```python
from build123d import *

# Parameters (mm, degrees)
SKETCH1_R                = 4
BOSS_EXTRUDE1_DEPTH      = 28
SKETCH2_W                = 40.5
SKETCH2_H                = 38
CUT_EXTRUDE1_DEPTH       = 23
SKETCH3_R                = 9.65
CUT_EXTRUDE2_DEPTH       = 5
CUT_EXTRUDE3_START       = -5
SKETCH4_R                = 9.65
CUT_EXTRUDE3_DEPTH       = 5
SKETCH8_R                = 1.15
CUT_EXTRUDE7_DEPTH       = 76.219678276
CHAMFER1_SIZE            = 23
CHAMFER1_SIZE2           = 43.5
SKETCH9_R                = 2.2
CUT_EXTRUDE8_DEPTH       = 97.701654612
CUT_EXTRUDE9_DEPTH       = 3
CUT_EXTRUDE9_DEPTH_BACK  = 4
CHAMFER2_SIZE            = 3
SKETCH15_R               = 1.7
CUT_EXTRUDE11_DEPTH      = 76.219678334
SKETCH16_W               = 26
SKETCH16_H               = 38
CUT_EXTRUDE12_DEPTH      = 67.075411499
FILLET6_R                = 1.5
CUT_EXTRUDE13_START      = -17
CUT_EXTRUDE13_DEPTH      = 17
BOSS_EXTRUDE3_DEPTH      = 4.5
BOSS_EXTRUDE3_DEPTH_BACK = 4.5
SKETCH21_R               = 1.65
SKETCH22_R               = 4.5
CUT_EXTRUDE14_DEPTH      = 7
CHAMFER4_SIZE            = 8.5
CHAMFER4_SIZE2           = 10
FILLET1_R                = 5
FILLET2_R                = 6
FILLET4_R                = 12
CUT_EXTRUDE15_DEPTH      = 3.8
CUT_EXTRUDE18_REACH      = 77.22
SKETCH26_R               = 3.15


with BuildPart() as part:
    # Sketch1 → Boss-Extrude1 (new body)
    with BuildSketch(Plane.XY):
        with BuildLine():
            Line((-55, -23.6), (34.5, -23.6))
            Line((34.5, -23.6), (34.5, 19.4))
            Line((34.5, 19.4), (-28.5, 19.4))
            Line((-28.5, 19.4), (-28.5, 12.180409823))
            ThreePointArc((-28.5, 12.180409823), (-20.217668105, -2.285689125), (-33, -12.985083113))
            Line((-33, -12.985083113), (-36, -12.985083113))
            ThreePointArc((-36, -12.985083113), (-41.689100041, -11.672468641), (-46.228019527, -8))
            Line((-46.228019527, -8), (-55, -8))
            Line((-55, -8), (-55, -23.6))
        make_face()
        Circle(SKETCH1_R, mode=Mode.SUBTRACT)
        with BuildLine():
            Line((-23, 11.35), (-20, 11.35))
            ThreePointArc((-20, 11.35), (-18.35, 13), (-20, 14.65))
            Line((-20, 14.65), (-23, 14.65))
            ThreePointArc((-23, 14.65), (-24.65, 13), (-23, 11.35))
        make_face(mode=Mode.SUBTRACT)
        with BuildLine():
            Line((-23, -14.65), (-20, -14.65))
            ThreePointArc((-20, -14.65), (-18.35, -13), (-20, -11.35))
            Line((-20, -11.35), (-23, -11.35))
            ThreePointArc((-23, -11.35), (-24.65, -13), (-23, -14.65))
        make_face(mode=Mode.SUBTRACT)
        with BuildLine():
            Line((-46, -11.35), (-49, -11.35))
            ThreePointArc((-49, -11.35), (-50.65, -13), (-49, -14.65))
            Line((-49, -14.65), (-46, -14.65))
            ThreePointArc((-46, -14.65), (-44.35, -13), (-46, -11.35))
        make_face(mode=Mode.SUBTRACT)
    extrude(amount=BOSS_EXTRUDE1_DEPTH)

    # Sketch2 → Cut-Extrude1 (cut)
    with BuildSketch(Plane.XY.offset(28)):
        with Locations((-34.75, 0.4)):
            Rectangle(SKETCH2_W, SKETCH2_H)
    extrude(amount=-CUT_EXTRUDE1_DEPTH, mode=Mode.SUBTRACT)

    # Sketch3 → Cut-Extrude2 (cut)
    with BuildSketch(Plane.XY.offset(28)):
        Circle(SKETCH3_R)
    extrude(amount=-CUT_EXTRUDE2_DEPTH, mode=Mode.SUBTRACT)

    # Sketch4 → Cut-Extrude3 (cut)
    with BuildSketch(Plane(origin=(0, 0, 0), x_dir=(-1, 0, 0), z_dir=(0, 0, -1)).offset(CUT_EXTRUDE3_START)):
        with Locations(Location((0, 0, 0), (0, 0, 180))):
            Circle(SKETCH4_R)
    extrude(amount=CUT_EXTRUDE3_DEPTH, mode=Mode.SUBTRACT)

    # Sketch8 → Cut-Extrude7 (cut, through all)
    with BuildSketch(Plane.XZ.offset(23.6)):
        with Locations(Location((3.375, 15.5, 0), (0, 0, 270))):
            Circle(SKETCH8_R)
    extrude(amount=-CUT_EXTRUDE7_DEPTH, mode=Mode.SUBTRACT)

    # Chamfer1
    chamfer1_edges = [part.edges().sort_by_distance(p)[0] for p in [
        (-55, -21.1, 28),
    ]]
    chamfer1_side = [part.faces().sort_by_distance(p)[0] for p in [
        (-55, -18.958031088, 10.841968912),
    ]]
    chamfer(chamfer1_edges, length=CHAMFER1_SIZE, length2=CHAMFER1_SIZE2, reference=chamfer1_side[0])

    # Sketch9 → Cut-Extrude8 (cut, through all)
    with BuildSketch(Plane(origin=(34.5, 0, 0), x_dir=(0, 0, -1), z_dir=(1, 0, 0))):
        with Locations((-8, 13)):
            Circle(SKETCH9_R)
        with Locations((-23, 13)):
            Circle(SKETCH9_R)
    extrude(amount=-CUT_EXTRUDE8_DEPTH, mode=Mode.SUBTRACT)

    # Sketch10 → Cut-Extrude9 (cut, two sides: drawn at the far end of the back side and taken through both)
    with BuildSketch(Plane.ZY.offset(14.5).offset(-CUT_EXTRUDE9_DEPTH_BACK)):
        Polygon((5.1, 14.674315781), (5.1, 11.325684219), (8, 9.651368439), (10.9, 11.325684219), (10.9, 14.674315781), (8, 16.348631561), align=None)
        Polygon((25.9, 11.325684219), (25.9, 14.674315781), (23, 16.348631561), (20.1, 14.674315781), (20.1, 11.325684219), (23, 9.651368439), align=None)
    extrude(amount=CUT_EXTRUDE9_DEPTH + CUT_EXTRUDE9_DEPTH_BACK, mode=Mode.SUBTRACT)

    # Chamfer2
    chamfer2_edges = [part.edges().sort_by_distance(p)[0] for p in [
        (-14.5, -18.6, 15.706896552),
    ]]
    chamfer(chamfer2_edges, length=CHAMFER2_SIZE)

    # Sketch15 → Cut-Extrude11 (cut, through all)
    with BuildSketch(Plane.XZ.offset(23.6)):
        with Locations(Location((-20.625, 15, 0), (0, 0, 270))):
            Circle(SKETCH15_R)
        with Locations(Location((29.375, 15, 0), (0, 0, 270))):
            Circle(SKETCH15_R)
    extrude(amount=-CUT_EXTRUDE11_DEPTH, mode=Mode.SUBTRACT)

    # Sketch16 → Cut-Extrude12 (cut, through all)
    with BuildSketch(Plane.XY.offset(28)):
        with Locations((21.5, 0.4)):
            Rectangle(SKETCH16_W, SKETCH16_H)
    extrude(amount=-CUT_EXTRUDE12_DEPTH, mode=Mode.SUBTRACT)

    # Fillet6
    fillet6_edges = [part.edges().sort_by_distance(p)[0] for p in [
        (8.5, -18.6, 14),
    ]]
    fillet(fillet6_edges, radius=FILLET6_R)

    # Sketch17 → Cut-Extrude13 (cut)
    with BuildSketch(Plane.XY.offset(28).offset(CUT_EXTRUDE13_START)):
        with BuildLine():
            Line((0, 4), (0, 15.733500455))
            Line((0, 15.733500455), (8.5, 15.733500455))
            Line((8.5, 15.733500455), (8.5, -8.907477288))
            Line((8.5, -8.907477288), (0, -4))
            ThreePointArc((0, -4), (4, 0), (0, 4))
        make_face()
    extrude(amount=CUT_EXTRUDE13_DEPTH, mode=Mode.SUBTRACT)

    # Sketch20 → Cut-Revolve1 (revolve, cut)
    with BuildSketch(Plane.XY.offset(15.5), mode=Mode.PRIVATE) as cut_revolve1_sk:
        Polygon((3.375, -11.8), (7.375, -3.8), (3.375, -3.8), align=None)
    revolve(cut_revolve1_sk.sketch.rotate(Axis((3.375, -3.8, 15.5), (0, -1, 0)), 270), axis=Axis((3.375, -3.8, 15.5), (0, -1, 0)), mode=Mode.SUBTRACT)

    # Sketch21 → Boss-Extrude3 (add, two sides: drawn at the far end of the back side and taken through both)
    with BuildSketch(Plane.XY.offset(15.5).offset(-BOSS_EXTRUDE3_DEPTH_BACK)):
        with BuildLine():
            Line((14.782175503, -11.85318602), (7.25, -8.185789452))
            Line((7.25, -8.185789452), (7.25, -18.6))
            Line((7.25, -18.6), (21.799747468, -18.6))
            Line((21.799747468, -18.6), (15.724873734, -12.525126266))
            ThreePointArc((15.724873734, -12.525126266), (15.281498664, -12.14990997), (14.782175503, -11.85318602))
        make_face()
        with Locations((13.25, -15)):
            Circle(SKETCH21_R, mode=Mode.SUBTRACT)
    extrude(amount=BOSS_EXTRUDE3_DEPTH + BOSS_EXTRUDE3_DEPTH_BACK)

    # Sketch22 → Cut-Extrude14 (cut)
    with BuildSketch(Plane.XY.offset(20)):
        with Locations((13.25, -15)):
            Circle(SKETCH22_R)
    cut_extrude14 = extrude(amount=CUT_EXTRUDE14_DEPTH, mode=Mode.SUBTRACT)

    # Mirror1: Cut-Extrude14 across plane
    add(cut_extrude14.mirror(Plane.XY.offset(15.5)), mode=Mode.SUBTRACT)

    # Chamfer4
    chamfer4_edges = [part.edges().sort_by_distance(p)[0] for p in [
        (8.5, 17.566750228, 28),
    ]]
    chamfer4_side = [part.faces().sort_by_distance(p)[0] for p in [
        (7.87031754, -13.003738644, 28),
    ]]
    chamfer(chamfer4_edges, length=CHAMFER4_SIZE, length2=CHAMFER4_SIZE2, reference=chamfer4_side[0])

    # Fillet1
    fillet1_edges = [part.edges().sort_by_distance(p)[0] for p in [
        (-28.5, 19.4, 2.5),
    ]]
    fillet(fillet1_edges, radius=FILLET1_R)

    # Fillet2
    fillet2_edges = [part.edges().sort_by_distance(p)[0] for p in [
        (-55, -8, 2.5),
    ]]
    fillet(fillet2_edges, radius=FILLET2_R)

    # Fillet4
    fillet4_edges = [part.edges().sort_by_distance(p)[0] for p in [
        (34.5, -21.1, 28),
    ]]
    fillet(fillet4_edges, radius=FILLET4_R)

    # Sketch23 → Cut-Extrude15 (cut)
    with BuildSketch(Plane.XZ.offset(18.6)):
        Polygon((-0.775, 28.722034997), (7.525, 28.722034997), (7.525, 13.103996383), (3.375, 10.707992766), (-0.775, 13.103996383), align=None)
    extrude(amount=-CUT_EXTRUDE15_DEPTH, mode=Mode.SUBTRACT)

    # Sketch26 → Cut-Extrude18 (cut, up to next)
    with BuildSketch(Plane.XZ.offset(23.6), mode=Mode.PRIVATE) as cut_extrude18_sk1:
        with Locations(Location((3.375, 15.5, 0), (0, 0, 270))):
            Circle(SKETCH26_R)
    cut_extrude18_tool1 = extrude(cut_extrude18_sk1.sketch, amount=-CUT_EXTRUDE18_REACH, mode=Mode.PRIVATE) & part.part
    add(cut_extrude18_tool1.solids().sort_by_distance((3.375, -23.6, 15.5))[0], mode=Mode.SUBTRACT)


solid = part.part
```
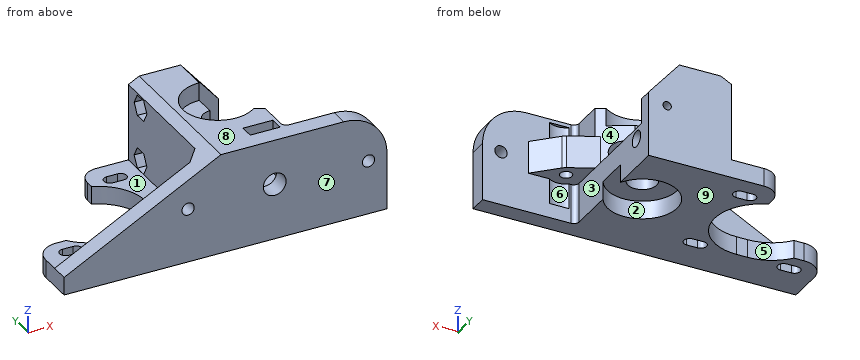
Design review of the part built by this model. Coordinates are the model's own, in mm. Face numbers are marked on the shaded views. A direction names the side the tool comes from. Give positions to 0.01 mm unless a question says otherwise; leave off trailing zeros. Loops run counter-clockwise (first coordinate to the right, second up) from the corner with the lowest first, then second, coordinate; pieces in that order, holes last. Notation, with made-up numbers: (54.25, 14.25) -> (104.25, 14.25) arc R21 ccw to (104.25, 31.25) -> close; hole circle Ø10 at (-27, 17.5). An arc over 180 degrees is marked (long way). One line per item, written item: value.
Q1. For pin 1 Ø2.5 at (x, z) = (-34.5, 3) entering from +Y; pin 2 Ø10 at (x, y) = (-22, 10) entering from +Z; pin 3 Ø2 at (x, z) = (3.375, 15.5) entering from +Y; pin 4 Ø5 at (x, y) = (0, 7) entering from -Z, all flat-tipped, find the tip position at first contact; note any pin that passes through.
Numbers:
pin 1: stops at y = -12.99
pin 2: stops at z = 5
pin 3: passes through
pin 4: stops at z = 5
Q2. We need section C-C on x = -43. Give the boundary of the cut face in (y, z).
Numbers:
outline: (-23.6, 0) -> (-10.94, 0) -> (-10.94, 5) -> (-18.6, 5) -> (-18.6, 11.34) -> (-23.6, 11.34) -> close
Q3. We need section B-B on y = 2. Give the boundary of the cut face in (x, z).
Numbers:
outline: (-20.17, 0) -> (-9.44, 0) -> (-9.44, 5) -> (-3.46, 5) -> (-3.46, 23) -> (-9.44, 23) -> (-9.44, 28) -> (-11.5, 28) -> (-14.5, 26.41) -> (-14.5, 5) -> (-20.17, 5) -> close; (3.46, 5) -> (8.5, 5) -> (8.5, 11) -> (3.46, 11) -> close
Q4. Machinability: for the marked faces 1, 2, 3, 4 and 5, which of the approach directions +Z, -Z, +X, -X, +Y, -Y give a long, thin tool a straight path to every point of the face, cutting with its end or side? Answer none if there is none.
Numbers:
face 1: +Z, -X, +Y
face 2: -Z
face 3: -Z, +X, +Y
face 4: +Z, +X
face 5: +Z, -Z, +Y
Q5. We need section A-A on x = 13.25. Give the boundary of the cut face in (y, z), and give its area (3 significant figures).
Numbers:
outline: (-23.6, 0) -> (-18.6, 0) -> (-18.6, 4) -> (-19.5, 4) -> (-19.5, 11) -> (-16.65, 11) -> (-16.65, 20) -> (-19.5, 20) -> (-19.5, 27) -> (-18.6, 27) -> (-18.6, 28) -> (-23.6, 28) -> close; (-13.35, 11) -> (-11.11, 11) -> (-11.11, 20) -> (-13.35, 20) -> close
area: 165 mm^2
Q6. Draft analysis for pull direction Z (two halves, no side actions). For the marked faces 6, 7, 8 and 9, state which applies: pulls with the +Z half, pulls with the -Z half, needs draft (parallel to the pull), parting line crosses it, or undercut.
Numbers:
face 6: undercut
face 7: needs draft
face 8: pulls with the +Z half
face 9: pulls with the -Z half
Q7. We need section D-D on x = 25.5. Give the boundary of the cut face in (y, z), and give its area (3 significant figures).
Numbers:
outline: (-23.6, 0) -> (-18.6, 0) -> (-18.6, 27.62) -> (-23.6, 27.62) -> close
area: 138 mm^2
Q8. For L1, parallel to Y at x = -1, z = 8; L2, parallel to Y at x = 26.5, z = 1; L3, parallel to Y at x = -10, z = 8.75, list the stretches that pass through material, from the lowest coordinate up.
Numbers:
L1: y = -23.6 to -3.87, 3.87 to 10.8, 15.2 to 19.4
L2: y = -23.6 to -18.6
L3: y = -23.6 to 10.93, 15.07 to 19.4
